Verification items for the finished model (mm, model axes). A direction names the side the tool comes from. Give positions to 0.01 mm unless a question says otherwise; leave off trailing zeros. Order: outer loops, then holes, each group sorted by start corner. A loop starts at its lowest first (then second) coordinate and runs counter-clockwise, first axis right, second up. Notation, with made-up numbers: (60, -23.5) -> (119, -23.5) arc R17 ccw to (119, -7.5) -> close; hole circle Ø10 at (15.25, -26.5). An arc over 180 degrees is marked (long way). One line per question, with ' | ' between items. Start each with the question number.
Q1. Mould release check, pull along Y, two halves, no side actions. Record for faces 3 (the flat face through (1, -1, 12)), 4 (the conical face through (2.05, -1.19, 11.88)), 5 (the cylindrical face through (-0.27, -1.22, 9.78)), 6 (the conical face through (2.05, 1.19, 3.62)): released by +Y, released by -Y, zero draft, split by the parting line, or undercut.
Q2. Access from +Z, -Z, +X, -X, +Y, -Y to the whole of each face (thin tool, end or side, straight path). Record for faces 1 (the flat face through (1.109, -1.958, 7.69)), 2 (the cylindrical face through (0, -1, 2)).
Q3. Section check B-B on z = 6.5. Record the cut outline in (x, y), plus the area to 3 significant figures.
Q4. Section check C-C on z = 1. Record the cut outline in (x, y), plus the area to 3 significant figures.
Q5. Material ranges on probe 1 along Y at (x, z) = (-0.6, 5.75); probe 2 along Z at (x, y) = (-0.05, -0.4); probe 3 along X at (y, z) = (-0.5, 9.75), recorded low to high. Write a range as [from, to].
Q6. Go/stop test with flat-tipped pins: pin 1 (1 mm diameter, centred on y = 0.5, z = 2.5, fed in from -X); pin 2 (2 mm diameter, centred on x = 1.5, z = 9.5, fed in from -Y). Record where each tip stops, or that it passes through.
Q7. Section check A-A on z = 9. Record the cut outline in (x, y).
from build123d import *

# Parameters (mm, degrees)
SKETCH1_R           = 1
BOSS_EXTRUDE1_DEPTH = 3.5
BOSS_EXTRUDE2_DEPTH = 8.5
SKETCH3_R           = 1.25
CUT_EXTRUDE1_DEPTH  = 4.5
SKETCH4_OUTSIDE_W   = 36.23
SKETCH4_OUTSIDE_H   = 36.926
SKETCH4_OUTSIDE_R   = 2.25
CUT_EXTRUDE2_DEPTH  = 13.482487733
CUT_EXTRUDE2_DRAFT  = -45
SKETCH6_OUTSIDE_W   = 29.602
SKETCH6_OUTSIDE_H   = 30.298
SKETCH6_OUTSIDE_R   = 2.25
CUT_EXTRUDE3_DEPTH  = 10.16856041
CUT_EXTRUDE3_DRAFT  = -45


with BuildPart() as part:
    # Sketch1 → Boss-Extrude1 (new body)
    with BuildSketch(Plane.XY):
        Circle(SKETCH1_R)
    extrude(amount=BOSS_EXTRUDE1_DEPTH)

    # Sketch2 → Boss-Extrude2 (add)
    with BuildSketch(Plane.XY.offset(3.5)):
        Polygon((0, 2.598076211), (-2.25, 1.299038106), (-2.25, -1.299038106), (0, -2.598076211), (2.25, -1.299038106), (2.25, 1.299038106), align=None)
    extrude(amount=BOSS_EXTRUDE2_DEPTH)

    # Sketch3 → Cut-Extrude1 (cut)
    with BuildSketch(Plane.XY.offset(12)):
        Circle(SKETCH3_R)
    extrude(amount=-CUT_EXTRUDE1_DEPTH, mode=Mode.SUBTRACT)


with BuildPart() as cut_extrude2_tool:
    # Sketch4 outside → Cut-Extrude2 (with draft: the straight prism first)
    with BuildSketch(Plane.XY.offset(12)):
        Rectangle(SKETCH4_OUTSIDE_W, SKETCH4_OUTSIDE_H)
        Circle(SKETCH4_OUTSIDE_R, mode=Mode.SUBTRACT)
    extrude(amount=-CUT_EXTRUDE2_DEPTH)
    # Cut-Extrude2: the draft: its side faces are tilted about the plane it starts from
    cut_extrude2_sides = [cut_extrude2_tool.faces().sort_by_distance(p)[0] for p in [
        (0, -18.463, 5.258756134),
        (18.115, 0, 5.258756134),
        (0, 18.463, 5.258756134),
        (-18.115, 0, 5.258756134),
        (-2.25, 0, 5.258756134),
    ]]
    draft(cut_extrude2_sides, Plane.XY.offset(12), CUT_EXTRUDE2_DRAFT)


with BuildPart() as part_1:
    add(part.part)

    # Cut-Extrude2: cut by cut_extrude2_tool
    add(cut_extrude2_tool.part, mode=Mode.SUBTRACT)


with BuildPart() as cut_extrude3_tool:
    # Sketch6 outside → Cut-Extrude3 (with draft: the straight prism first)
    with BuildSketch(Plane(origin=(0, 0, 3.5), x_dir=(-1, 0, 0), z_dir=(0, 0, -1))):
        Rectangle(SKETCH6_OUTSIDE_W, SKETCH6_OUTSIDE_H)
        Circle(SKETCH6_OUTSIDE_R, mode=Mode.SUBTRACT)
    extrude(amount=-CUT_EXTRUDE3_DEPTH)
    # Cut-Extrude3: the draft: its side faces are tilted about the plane it starts from
    cut_extrude3_sides = [cut_extrude3_tool.faces().sort_by_distance(p)[0] for p in [
        (0, -15.149, 8.584280205),
        (-14.801, 0, 8.584280205),
        (0, 15.149, 8.584280205),
        (14.801, 0, 8.584280205),
        (2.25, 0, 8.584280205),
    ]]
    draft(cut_extrude3_sides, Plane(origin=(0, 0, 3.5), x_dir=(-1, 0, 0), z_dir=(0, 0, -1)), CUT_EXTRUDE3_DRAFT)


with BuildPart() as part_2:
    add(part_1.part)

    # Cut-Extrude3: cut by cut_extrude3_tool
    add(cut_extrude3_tool.part, mode=Mode.SUBTRACT)


solid = part_2.part
Filled in:
1) face 3: zero draft | face 4: released by -Y | face 5: undercut | face 6: released by +Y
2) face 1: +Z, -Z, +X, -Y | face 2: -Z
3) outline: (-2.25, -1.3) -> (0, -2.6) -> (2.25, -1.3) -> (2.25, 1.3) -> (0, 2.6) -> (-2.25, 1.3) -> close | area: 17.5 mm²
4) outline: circle Ø2 at (0, 0) | area: 3.14 mm²
5) probe 1: [-2.25, 2.25] | probe 2: [0, 7.5] | probe 3: [-2.25, -1.15], [1.15, 2.25]
6) pin 1: x = -1 | pin 2: y = -2.31
7) outline: (-2.25, -1.3) -> (0, -2.6) -> (2.25, -1.3) -> (2.25, 1.3) -> (0, 2.6) -> (-2.25, 1.3) -> close; hole circle Ø2.5 at (0, 0)
